Part model, mm, in its own coordinate system. A direction names the side the tool comes from. Round coordinates to 2 decimals unless told otherwise and drop trailing zeros. Loops run counter-clockwise (first coordinate to the right, second up) from the corner with the lowest first, then second, coordinate; pieces in that order, holes last.
(1) Cut at D-D on x = 84. List the corners of the cut face in (y, z) (3 decimals), then the cut area to 3 significant figures.
(2) Tool access for faces 4 (the face through (146.046, 0.583, 2.191)), 5 (the face through (17.579, -55.387, 2.191)), 6 (the face through (109.234, 23.811, 2.254)): list every direction of +Z, -Z, +X, -X, +Y, -Y with a clear straight run to the whole face (end or side of a thin tool).
(3) Flat gauge pins, fed straight in: pin 1 (7.5 mm diameter, centred on x = 0, y = -45, fed in from -Z); pin 2 (11 mm diameter, centred on x = 114.3, y = -42.6, fed in from +Z) (3 decimals); pin 3 (1.5 mm diameter, centred on y = -21.5, z = 2, fed in from -X); pin 4 (1.3 mm diameter, centred on x = 117.5, z = 3, fed in from -Y). Where does each tip first touch, or does it go through?
(4) Cut at B-B on y = 0. List the corners of the cut face in (x, z) (3 decimals).
(5) Probe probe 1 along Y at (x, z) = (44.45, 3.2); probe 2 along Y at (x, z) = (-31.75, 1.4); probe 3 along Y at (x, z) = (0, 2.1). List the from-to ranges inside material, lowest first.
(6) Mould opens along Y. For faces 1 (the face through (43, 1, 4.445)), 2 (the face through (117, -20.972, 2)), 3 (the face through (46.024, -63.002, 2.191)) say: +Y half, -Y half, draft (parallel to the pull), parting line (faces both ways), or undercut.
(7) Cut at A-A on x = 44.45. List the corners of the cut face in (y, z) (3 decimals), then the cut area to 3 significant figures.
(8) Cut at C-C on x = 0. List the corners of the cut face in (y, z) (3 decimals), then the cut area to 3 significant figures.
Autodesk Inventor part; units mm, degrees
ref_plane "YZ Plane" through (0, 0, 0) normal (1, 0, 0) x (0, 1, 0)
ref_plane "XZ Plane" through (0, 0, 0) normal (0, 1, 0) x (-1, 0, 0)
ref_plane "XY Plane" through (0, 0, 0) normal (0, 0, 1) x (1, 0, 0)
sketch "Boceto1" plane through (0, 0, 0) normal (0, 0, 1) x (1, 0, 0)
  circle A0 centre (0, 0) radius 57.15
  circle A1 centre (101.6, 0) radius 44.45
  circle A2 centre (-31.75, 47.519) radius 11.1125
  circle A3 centre (-31.75, -47.519) radius 11.1125
  circle A4 centre (114.3, 42.5971) radius 11.1125
  circle A5 centre (114.3, -42.5971) radius 11.1125
  line L0 (7.1437, 56.7018) -> (107.1562, 44.1014)
  circle A6 centre (44.45, 52.0016) radius 11.1125
  line L1 (7.1437, -56.7018) -> (107.1562, -44.1014)
  circle A7 centre (44.45, -52.0016) radius 11.1125
  dimension "d0" = 114.3
  dimension "d1" = 88.9
  dimension "d2" = 203.2
  dimension "d3" = 22.225
  dimension "d4" = 22.225
  dimension "d7" = 22.225
  dimension "d8" = 22.225
  dimension "d11" = 22.225
  dimension "d13" = 0
  dimension "d14" = 22.225
  dimension "d27" = 12.7
  dimension "d28" = 12.7
  dimension "d29" = 44.45
  dimension "d30" = 44.45
  dimension "d31" = 31.75
  dimension "d32" = 31.75
extrude "Extrusión1" add sketch "Boceto1" along normal blind 4.445
sketch "Boceto2" plane through (0, 0, 4.445) normal (0, 0, 1) x (1, 0, 0)
  arc A0 (-21.9537, 52.7651) -> (-40.3458, 40.4764) centre (-31.75, 47.519) ccw
  circle A1 centre (-31.75, 47.519) radius 4.7625
  arc A2 (-40.3458, -40.4764) -> (-21.9537, -52.7651) centre (-31.75, -47.519) ccw
  circle A3 centre (-31.75, -47.519) radius 4.7625
  arc A4 (33.4247, -53.3907) -> (55.4753, -50.6125) centre (44.45, -52.0016) ccw
  circle A5 centre (44.45, -52.0016) radius 4.7625
  arc A6 (55.4753, 50.6125) -> (33.4247, 53.3907) centre (44.45, 52.0016) ccw
  circle A7 centre (44.45, 52.0016) radius 4.7625
  arc A8 (124.4689, 38.1158) -> (103.3657, 44.5789) centre (114.3, 42.5971) ccw
  circle A9 centre (114.3, 42.5971) radius 4.7625
  arc A10 (103.3657, -44.5789) -> (124.4689, -38.1158) centre (114.3, -42.5971) ccw
  circle A11 centre (114.3, -42.5971) radius 4.7625
  point P0 (0, 0)
  dimension "d18" = 9.525
  dimension "d19" = 9.525
  dimension "d20" = 9.525
  dimension "d21" = 9.525
  dimension "d22" = 9.525
  dimension "d23" = 9.525
extrude "Extrusión2" cut sketch "Boceto2" against normal up to surface (4.445 mm away)
fillet "Empalme1" radius 6.35 12 edges at (-21.9537, -52.7651, 2.2225) (-40.3458, -40.4764, 2.2225) (33.4247, -53.3907, 2.2225) (55.4753, -50.6125, 2.2225) (124.4689, -38.1158, 2.2225) (-40.3458, 40.4764, 2.2225) (-21.9537, 52.7651, 2.2225) (33.4247, 53.3907, 2.2225) (55.4753, 50.6125, 2.2225) (103.3657, 44.5789, 2.2225) (124.4689, 38.1158, 2.2225) (103.3657, -44.5789, 2.2225)
sketch "Boceto3" plane through (0, 0, 0) normal (0, 0, -1) x (-1, 0, 0)
  circle A0 centre (0, 0) radius 7.1437
  circle A1 centre (0, -45) radius 6.35
  circle A2 centre (0, 45) radius 6.35
  line L0 (0, -45) -> (0, 0)
  line L1 (0, 0) -> (0, 45)
  dimension "d33" = 14.2875
  dimension "d34" = 12.7
  dimension "d35" = 12.7
  dimension "d36" = 45
  dimension "d37" = 45
extrude "Extrusión3" cut sketch "Boceto3" against normal up to surface (4.445 mm away)
sketch "Boceto4" plane through (0, 0, 4.445) normal (0, 0, 1) x (1, 0, 0)
  circle A0 centre (93.4212, 0) radius 6.35
  line L0 (65.4212, -28) -> (121.4212, -28)
  line L1 (121.4212, -28) -> (121.4212, 28)
  line L2 (121.4212, 28) -> (65.4212, 28)
  line L3 (65.4212, 28) -> (65.4212, -28)
  line L4 (69.6712, -23.75) -> (117.1712, -23.75)
  line L5 (117.1712, -23.75) -> (117.1712, 23.75)
  line L6 (117.1712, 23.75) -> (69.6712, 23.75)
  line L7 (69.6712, 23.75) -> (69.6712, -23.75)
  circle A1 centre (74.8306, -23.75) radius 2.7781
  circle A2 centre (112.0118, -23.75) radius 2.7781
  circle A3 centre (122.3306, -23.75) radius 2.7781
  circle A4 centre (64.5118, -23.75) radius 2.7781
  line L8 (64.5118, -26.5281) -> (74.8306, -26.5281)
  line L9 (64.5118, -20.9719) -> (74.8306, -20.9719)
  line L10 (112.0118, -26.5281) -> (122.3306, -26.5281)
  line L11 (122.3306, -20.9719) -> (112.0118, -20.9719)
  circle A5 centre (74.8306, 23.75) radius 2.7781
  circle A6 centre (64.5118, 23.75) radius 2.7781
  line L12 (64.5118, 20.9719) -> (74.8306, 20.9719)
  line L13 (64.5118, 26.5281) -> (74.8306, 26.5281)
  circle A7 centre (112.0118, 23.75) radius 2.7781
  circle A8 centre (122.3306, 23.75) radius 2.7781
  line L14 (112.0118, 20.9719) -> (122.3306, 20.9719)
  line L15 (112.0118, 26.5281) -> (122.3306, 26.5281)
  circle A9 centre (98.5806, 0) radius 6.35
  circle A10 centre (88.2618, 0) radius 6.35
  line L16 (98.5806, 6.35) -> (88.2618, 6.35)
  line L17 (98.5806, -6.35) -> (88.2618, -6.35)
  point P0 (0, 0)
  dimension "d40" = 12.7
  dimension "d41" = 56
  dimension "d42" = 56
  dimension "d43" = 28
  dimension "d44" = 28
  dimension "d45" = 0
  dimension "d46" = 93.4212
  dimension "d47" = 47.5
  dimension "d48" = 47.5
  dimension "d49" = 23.75
  dimension "d50" = 23.75
  dimension "d57" = 5.5563
  dimension "d58" = 5.1594
  dimension "d59" = 5.5563
  dimension "d60" = 5.5563
  dimension "d61" = 5.1594
  dimension "d62" = 5.1594
  dimension "d63" = 5.5563
  dimension "d64" = 5.1594
  dimension "d65" = 0
  dimension "d66" = 5.5563
  dimension "d67" = 5.5563
  dimension "d68" = 5.1594
  dimension "d69" = 5.1594
  dimension "d70" = 0
  dimension "d71" = 5.5563
  dimension "d72" = 5.5563
  dimension "d73" = 5.1594
  dimension "d74" = 5.1594
  dimension "d75" = 0
  dimension "d78" = 12.7
  dimension "d79" = 12.7
  dimension "d80" = 5.1594
  dimension "d81" = 5.1594
extrude "Extrusión4" cut sketch "Boceto4" against normal up to next contours A0 A9 A10 | A0 A9 | A9 A10 A0 | A0 L16 A9 | A9 L17 A0 | A0 A10 A9 | A0 A10 L16 | A10 A9 | A9 A10 A0 | L17 A10 A0 | A0 A10 | L8 A4 L3 | L3 A4 L9 L7 L4 A1 L8 | L10 A2 L4 L5 L11 L1 A3 | L1 A3 L10 | A4 L3 | L3 A4 | A1 L4 | A3 L1 | L1 A3 | A2 L4 | A4 L9 L3 | L4 A1 | L4 L7 L9 A1 | L1 L11 A3 | A2 L11 L5 L4 | L4 A2 | L12 A6 L3 | L3 A6 L13 A5 L6 L7 L12 | L14 L5 L6 A7 L15 L1 A8 | L1 A8 L14 | A6 L3 | L3 A6 | L7 L6 A5 L12 | A8 L1 | L1 A8 | L14 A7 L6 L5 | A6 L13 L3 | A5 L6 | L1 L15 A8 | A7 L6 | A5 L6 | L6 A7
equation "\"d16\" = t"
equation "\"d18\" = Q"
equation "\"d19\" = Q"
equation "\"d20\" = Q"
equation "\"d21\" = Q"
equation "\"d22\" = Q"
equation "\"d23\" = Q"
equation "\"d33\" = DF"
equation "\"d34\" = NF"
equation "\"d35\" = NF"
equation "\"d40\" = DM"
equation "\"d41\" = AM"
equation "\"d42\" = AM"
equation "\"d43\" = 0.5 * AM"
equation "\"d44\" = 0.5 * AM"
equation "\"d47\" = BM"
equation "\"d48\" = BM"
equation "\"d49\" = 0.5 * BM"
equation "\"d50\" = 0.5 * BM"
equation "\"d57\" = NM"
equation "\"d59\" = NM"
equation "\"d60\" = NM"
equation "\"d63\" = NM"
equation "\"d66\" = NM"
equation "\"d67\" = NM"
equation "\"d71\" = NM"
equation "\"d72\" = NM"
equation "\"d78\" = DM"
equation "\"d79\" = DM"
equation "\"t\" = 4.445"
equation "\"Q\" = 9.525"
equation "\"DF\" = 14.2875"
equation "\"NF\" = 12.7"
equation "\"DM\" = 12.7"
equation "\"NM\" = 5.55625"
equation "\"CM\" = 93.4212"
equation "\"AM\" = 56"
equation "\"BM\" = 47.5"
properties part number "SIDE REDUCTION PLATE I"
Final values:
1. outline: (-47.019, 0) - (-4.707, 0) - (-4.707, 4.445) - (-47.019, 4.445) - close; (4.707, 0) - (47.019, 0) - (47.019, 4.445) - (4.707, 4.445) - close
1. area: 376 mm2
2. face 4: +Z, -Z, +X
2. face 5: +Z, -Z, -Y
2. face 6: +Z, -Z
3. pin 1: passes through
3. pin 2: stops at z = 4.445
3. pin 3: stops at x = -53.25
3. pin 4: stops at y = -53.41
4. outline: (-57.15, 0) - (-7.144, 0) - (-7.144, 4.445) - (-57.15, 4.445) - close; (7.144, 0) - (81.912, 0) - (81.912, 4.445) - (7.144, 4.445) - close; (104.931, 0) - (146.05, 0) - (146.05, 4.445) - (104.931, 4.445) - close
5. probe 1: y = -63.11 to -56.76, -47.24 to 47.24, 56.76 to 63.11
5. probe 2: y = -58.63 to -52.28, -42.76 to 42.76, 52.28 to 58.63
5. probe 3: y = -57.15 to -51.35, -38.65 to -7.14, 7.14 to 38.65, 51.35 to 57.15
6. face 1: draft
6. face 2: undercut
6. face 3: -Y half
7. outline: (-63.114, 0) - (-56.764, 0) - (-56.764, 4.445) - (-63.114, 4.445) - close; (-47.239, 0) - (47.239, 0) - (47.239, 4.445) - (-47.239, 4.445) - close; (56.764, 0) - (63.114, 0) - (63.114, 4.445) - (56.764, 4.445) - close
7. area: 476 mm2
8. outline: (-57.15, 0) - (-51.35, 0) - (-51.35, 4.445) - (-57.15, 4.445) - close; (-38.65, 0) - (-7.144, 0) - (-7.144, 4.445) - (-38.65, 4.445) - close; (7.144, 0) - (38.65, 0) - (38.65, 4.445) - (7.144, 4.445) - close; (51.35, 0) - (57.15, 0) - (57.15, 4.445) - (51.35, 4.445) - close
8. area: 332 mm2
